The drawing under review shows one solid part. Ordinate dimensions are in mm from its lowest x, y, z. A direction names the side the tool comes from. Give positions to 0.01 mm unless a question says otherwise; leave off trailing zeros. Order: outer loops, then holes, each group sorted by start corner. A loop starts at its lowest first (then second) coordinate and runs counter-clockwise, first axis right, second up. Notation, with made-up numbers: (42, 60) -> (101, 60) arc R20 cw to (101, 73) -> close; hole circle Ø1 at (-21, 55). An arc over 180 degrees is marked (long way). One line per item, written item: value. Start each with the question number.
1) Wall thickness on line 1 along Y through (x, z) = (1.05, 5); line 2 along Z through (x, y) = (18, 2.2): over which ranges is each line inside the solid? List them lowest first. Write a range as from..to.
2) Consider section B-B (x = 18). State the section outline as (y, z) points.
3) Tool access review of the marked faces 1 and 2: name each direction out of +Z, -Z, +X, -X, +Y, -Y from which nothing blocks a thin tool from reaching the whole face with its end or side.
4) Consider section D-D (x = 2.5). State the section outline as (y, z) points, plus the area to 3 significant figures.
5) For pin 1 (4 mm diameter, centred on x = 6, y = 6, fed in from -Z); pin 2 (5 mm diameter, centred on y = 8, z = 15, fed in from +X); pin 3 (5 mm diameter, centred on y = 14, z = 13, fed in from +X); pin 4 (5 mm diameter, centred on x = 13, z = 8.5, fed in from +Y), all flat-tipped, find the tip position at first contact; note any pin that passes through.
6) Consider section A-A (z = 5). State how many separate pieces and enclosed holes the cut face has, plus the area to 3 significant figures.
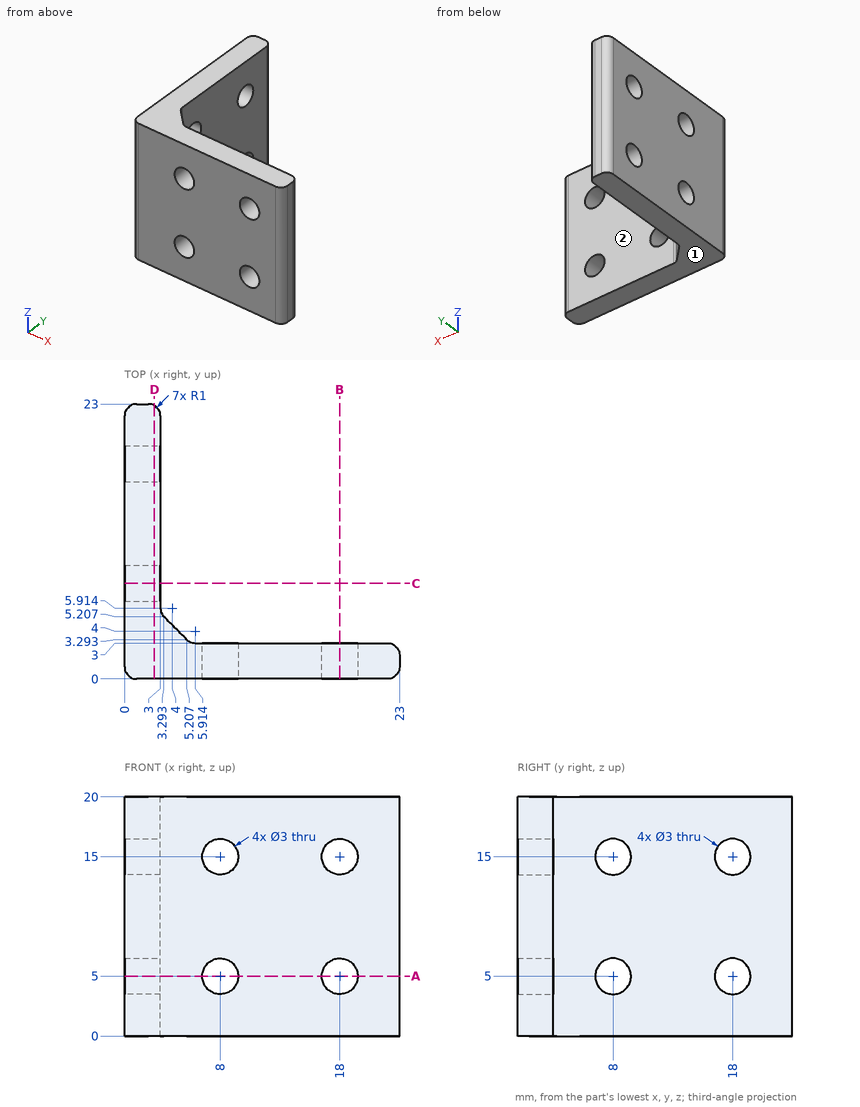
Checked values:
1. line 1: y = 0..6.5, 9.5..16.5, 19.5..23
1. line 2: z = 0..3.5, 6.5..13.5, 16.5..20
2. outline: (0, 0) -> (3, 0) -> (3, 3.5) -> (0, 3.5) -> close; (0, 6.5) -> (3, 6.5) -> (3, 13.5) -> (0, 13.5) -> close; (0, 16.5) -> (3, 16.5) -> (3, 20) -> (0, 20) -> close
3. face 1: -Z, +X, -X, +Y, -Y
3. face 2: +Z, -Z, +X, +Y
4. outline: (0, 0) -> (22.87, 0) -> (22.87, 20) -> (0, 20) -> close; hole circle Ø3 at (8, 5); hole circle Ø3 at (8, 15); hole circle Ø3 at (18, 5); hole circle Ø3 at (18, 15)
4. area: 429 mm^2
5. pin 1: passes through
5. pin 2: stops at x = 3.09
5. pin 3: stops at x = 3
5. pin 4: stops at y = 3
6. separate pieces: 5
6. enclosed holes: 0
6. area: 95.1 mm^2
